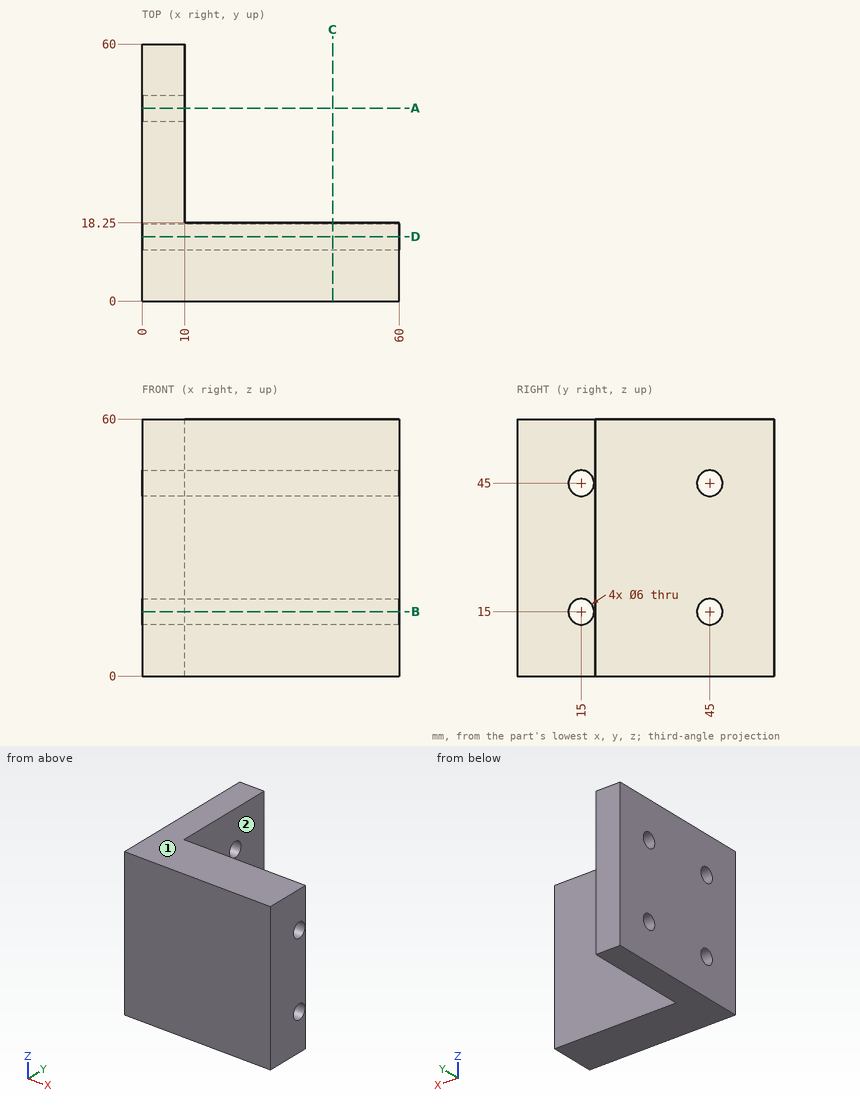
For this review, use the dimensioned drawing (mm, ordinates from the lowest corner) and the shaded views. A direction names the side the tool comes from. Give positions to 0.01 mm unless a question says otherwise; leave off trailing zeros. Order: outer loops, then holes, each group sorted by start corner. A loop starts at its lowest first (then second) coordinate and runs counter-clockwise, first axis right, second up.
1) Wall thickness on line 1 (Y direction, x = 44.5, z = 45); line 2 (Z direction, x = 6.5, y = 17); line 3 (Z direction, x = 15.5, y = 14.5): over which ranges is each line inside the solid? List them lowest first.
2) Take a section at C-C (x = 44.5). Give the boundary of the cut face in (y, z).
3) Take a section at B-B (z = 15). Give the boundary of the cut face in (x, y), then the cut area to 3 significant figures.
4) Take a section at A-A (y = 45). Give the boundary of the cut face in (x, z).
5) Insertion check: pin 1 (5.5 mm diameter, centred on y = 15, z = 45, fed in from -X); pin 2 (10 mm diameter, centred on x = 40, z = 32, fed in from -Y); pin 3 (1.5 mm diameter, centred on x = 34.5, z = 18.5, fed in from +Y); pin 4 (2 mm diameter, centred on y = 22.5, z = 31, fed in from +X). Each pin has a flat end and moves straight along its axis. Give the tip position at first contact, or say it passes through.
6) For the marked faces 1 and 2, list the 3-axis set-ups (+Z, -Z, +X, -X, +Y, -Y) from which the entire face can be reached by the end or side of a thin tool; tool diameter is ignored.
7) Take a section at D-D (y = 15). Give the boundary of the cut face in (x, z).
Derived:
1. line 1: y = 0 to 12, 18 to 18.25
1. line 2: z = 0 to 12.76, 17.24 to 42.76, 47.24 to 60
1. line 3: z = 0 to 12.04, 17.96 to 42.04, 47.96 to 60
2. outline: (0, 0) - (18.25, 0) - (18.25, 60) - (0, 60) - close; hole circle Ø6 at (15, 15); hole circle Ø6 at (15, 45)
3. outline: (0, 0) - (60, 0) - (60, 12) - (0, 12) - close; (0, 18) - (60, 18) - (60, 18.25) - (10, 18.25) - (10, 42) - (0, 42) - close; (0, 48) - (10, 48) - (10, 60) - (0, 60) - close
3. area: 1,090 mm2
4. outline: (0, 0) - (10, 0) - (10, 12) - (0, 12) - close; (0, 18) - (10, 18) - (10, 42) - (0, 42) - close; (0, 48) - (10, 48) - (10, 60) - (0, 60) - close
5. pin 1: passes through
5. pin 2: stops at y = 0
5. pin 3: stops at y = 18.25
5. pin 4: stops at x = 10
6. face 1: +Z, +X, -X, +Y, -Y
6. face 2: +Z, -Z, +X, +Y
7. outline: (0, 0) - (60, 0) - (60, 12) - (0, 12) - close; (0, 18) - (60, 18) - (60, 42) - (0, 42) - close; (0, 48) - (60, 48) - (60, 60) - (0, 60) - close
